The listing builds one solid part. Answer for the finished solid, in the listing's coordinates (mm). Give positions to 0.01 mm unless a question says otherwise; leave off trailing zeros. Order: outer loops, then holes, each group sorted by start corner. A loop starts at its lowest first (then second) coordinate and runs counter-clockwise, first axis right, second up.
```python
from build123d import *

# Parameters (mm, degrees)
SKETCH1_W                                      = 168.275
SKETCH1_H                                      = 168.275
BOSS_EXTRUDE1_DEPTH                            = 9.525
CBORE_FOR_8_SOCKET_HEAD_CAP_SCREW1_D           = 4.4958
CBORE_FOR_8_SOCKET_HEAD_CAP_SCREW1_CBORE_D     = 7.9375
CBORE_FOR_8_SOCKET_HEAD_CAP_SCREW1_CBORE_DEPTH = 4.1656
FILLET1_R                                      = 4.5212


with BuildPart() as part:
    # Sketch1 → Boss-Extrude1 (new body)
    with BuildSketch(Plane.XY):
        Rectangle(SKETCH1_W, SKETCH1_H)
    extrude(amount=BOSS_EXTRUDE1_DEPTH)

    # CBORE for #8 Socket Head Cap Screw1 (through all)
    with Locations(Plane.XY.offset(9.525)):
        with Locations((-79.629, 79.629), (0, 79.629), (79.629, 79.629), (79.629, 0), (0, -79.629), (79.629, -79.629), (-79.629, 0), (-79.629, -79.629)):
            CounterBoreHole(CBORE_FOR_8_SOCKET_HEAD_CAP_SCREW1_D / 2, CBORE_FOR_8_SOCKET_HEAD_CAP_SCREW1_CBORE_D / 2, CBORE_FOR_8_SOCKET_HEAD_CAP_SCREW1_CBORE_DEPTH)

    # Fillet1
    fillet1_edges = [part.edges().sort_by_distance(p)[0] for p in [
        (-84.1375, 84.1375, 4.7625),
        (84.1375, 84.1375, 4.7625),
        (84.1375, -84.1375, 4.7625),
        (-84.1375, -84.1375, 4.7625),
    ]]
    fillet(fillet1_edges, radius=FILLET1_R)


solid = part.part
```
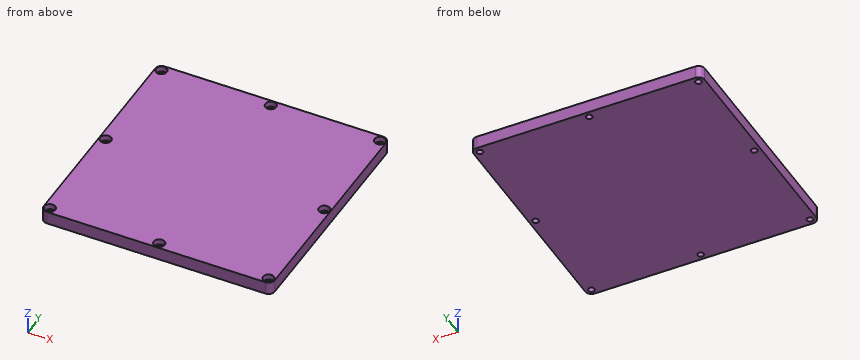
1) Given P1, Ø2.5, axis at x = 78.5, y = -79, coming from the +Z side; P2, Ø2.5, axis at x = 79.629, y = -79.629, coming from the -Z side, each flat-ended and moving along its own axis, determine where each tip first touches the part or whether it passes through.
Geometry says:
P1: stops at z = 5.36
P2: passes through
2) Straight lines are drawn through the part: probe 1 along Y at (x, z) = (0, 1.2); probe 2 along X at (y, z) = (2, 5.25); probe 3 along X at (y, z) = (-3, 8.5). For each, find the intervals that lie inside material, in ascending order.
Geometry says:
probe 1: y = -84.14 to -81.88, -77.38 to 77.38, 81.88 to 84.14
probe 2: x = -84.14 to -80.66, -78.6 to 78.6, 80.66 to 84.14
probe 3: x = -84.14 to -82.23, -77.03 to 77.03, 82.23 to 84.14
3) Find section A-A (x = 0). Write down the section's boundary in (y, z) (1 decimal), then the cut area to 3 significant figures.
Geometry says:
outline: (-84.1, 0) - (-81.9, 0) - (-81.9, 5.4) - (-83.6, 5.4) - (-83.6, 9.5) - (-84.1, 9.5) - close; (-77.4, 0) - (77.4, 0) - (77.4, 5.4) - (75.7, 5.4) - (75.7, 9.5) - (-75.7, 9.5) - (-75.7, 5.4) - (-77.4, 5.4) - close; (81.9, 0) - (84.1, 0) - (84.1, 9.5) - (83.6, 9.5) - (83.6, 5.4) - (81.9, 5.4) - close
area: 1,490 mm2
